Geometry check sheet. Reference: the model listing, model coordinates, mm. Face numbers are marked on the shaded views. A direction names the side the tool comes from. Give positions to 0.01 mm unless a question says otherwise; leave off trailing zeros. Order: outer loops, then holes, each group sorted by start corner. A loop starts at its lowest first (then second) coordinate and runs counter-clockwise, first axis right, second up. Notation, with made-up numbers: M 33,-31 L 78,-31 A21 cw 78,-17 Z; hole C 7.5,89.25 d8. An arc over 180 degrees is marked long. Answer as CSV lines item,"result". Start each with the question number.
Q1. Thickness scan on line 1 (X direction, y = 8, z = 3.75); line 2 (Y direction, x = -21, z = 3.25); line 3 (Y direction, x = -22.25, z = 1.6). Record the ranges inside material, lowest first.
Q2. Set-up check for the marked faces 1, 2, 3, 4 and 5: record each of +Z, -Z, +X, -X, +Y, -Y from which the full face is reachable in a straight line by a thin tool's end or side.
Q3. Section check C-C, the plane y = 9.5. Record the boundary of the cut face in (x, z) (3 decimals), then the cut area to 3 significant figures.
Q4. Section check A-A, the plane z = 2.85. Count the separate pieces of the cut face and the enclosed holes in it, then the cut area to 3 significant figures.
Q5. Section check B-B, the plane x = -19.25. Record the boundary of the cut face in (y, z) (3 decimals).
Q6. Mould release check, pull along X, two halves, no side actions. Record for the marked faces 6, 7 and 8: +X half, -X half, draft (parallel to the pull), parting line (faces both ways), or undercut.
Q7. Go/stop test with flat-tipped pins: pin 1 (0.6 mm diameter, centred on x = -26, z = 3.5, fed in from +Y); pin 2 (1 mm diameter, centred on x = -23.5, z = 3.5, fed in from -Y); pin 3 (1.5 mm diameter, centred on x = -18, y = 14.5, fed in from +Z) (3 decimals). Record where each tip stops, or that it passes through.
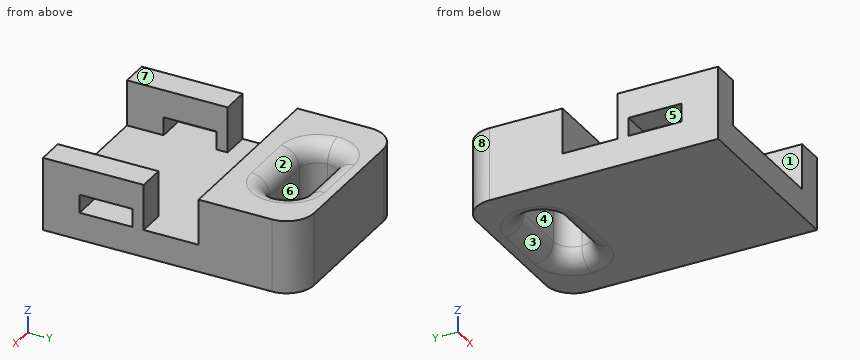
```python
from build123d import *

# Parameters (mm, degrees)
F0_W      = 12.7
F0_H      = 15.24
F1_DEPTH  = 5.08
F2_W      = 6.35
F2_H      = 2.54
F3_DEPTH  = 25.4
F4_R      = 1.26999
F5_R      = 1.905
F6_W      = 5.715
F6_H      = 1.27
F7_DEPTH  = 25.4
F8_W      = 8.89
F8_H      = 8.255
F9_DEPTH  = 3.175
F10_W     = 1.905
F10_H     = 3.81
F11_DEPTH = 1.905
F12_DEPTH = 2.54
F13_W     = 2.5417556653
F13_H     = 1.27
F14_DEPTH = 25.4
F15_W     = 1.905
F15_H     = 0.762
F16_DEPTH = 1.27
F17_W     = 1.905
F17_H     = 0.762
F18_DEPTH = 1.27


# Not quite as in the source:
# - a fillet or chamfer is up to 0.001 mm smaller than in the source, because OpenCascade refuses the exact size


with BuildPart() as f1:
    # F0 (on Top) → F1 (new body)
    with BuildSketch(Plane.XY):
        with Locations((-20.7207803614, 14.9625845535)):
            Rectangle(F0_W, F0_H)
    extrude(amount=F1_DEPTH)

    # F2 (on face) → F3 (cut)
    with BuildSketch(Plane.XY.offset(5.08)):
        with Locations((-20.7207803614, 19.4075845535)):
            Rectangle(F2_W, F2_H)
    extrude(amount=-F3_DEPTH, mode=Mode.SUBTRACT)

    # F4 (radius 1.27 in the source; OpenCascade refuses exactly that, so slightly less here)
    f4_edges = [f1.edges().sort_by_distance(p)[0] for p in [
        (-20.72078, 18.137585, 5.08),
        (-17.54578, 19.407585, 5.08),
        (-23.89578, 19.407585, 5.08),
        (-20.72078, 20.677585, 5.08),
        (-17.54578, 19.407585, 0),
        (-20.72078, 18.137585, 0),
        (-23.89578, 19.407585, 0),
        (-20.72078, 20.677585, 0),
        (-17.54578, 18.137585, 2.54),
        (-23.89578, 18.137585, 2.54),
        (-23.89578, 20.677585, 2.54),
        (-17.54578, 20.677585, 2.54),
    ]]
    fillet(f4_edges, radius=F4_R)

    # F5
    f5_edges = [f1.edges().sort_by_distance(p)[0] for p in [
        (-27.07078, 22.582585, 2.54),
        (-14.37078, 22.582585, 2.54),
    ]]
    fillet(f5_edges, radius=F5_R)

    # F6 (on face) → F7 (cut)
    with BuildSketch(Plane.YZ.offset(-14.3707803614)):
        with Locations((12.7400845535, 2.54)):
            Rectangle(F6_W, F6_H)
    extrude(amount=-F7_DEPTH, mode=Mode.SUBTRACT)

    # F8 (on face) → F9 (cut, through all)
    with BuildSketch(Plane.XY.offset(5.08)):
        with Locations((-20.7207803614, 11.4700845535)):
            Rectangle(F8_W, F8_H)
    extrude(amount=-F9_DEPTH, mode=Mode.SUBTRACT)

    # F10 (on face) → F11 (cut, through all)
    with BuildSketch(Plane.XY.offset(5.08)):
        with Locations((-26.1182803614, 13.6925845535)):
            Rectangle(F10_W, F10_H)
        with Locations((-15.3232803614, 13.6925845535)):
            Rectangle(F10_W, F10_H)
    extrude(amount=-F11_DEPTH, mode=Mode.SUBTRACT)

    # F12 (add): a face of the model
    f12_faces = [f1.faces().sort_by_distance(p)[0] for p in [
        (-20.7207803614, 7.3425845535, 1.7991666667),
    ]]
    extrude(f12_faces, amount=F12_DEPTH)

    # F13 (on face) → F14 (cut)
    with BuildSketch(Plane.YZ.offset(-14.3707803614)):
        with Locations((8.6117067208, 2.54)):
            Rectangle(F13_W, F13_H)
    extrude(amount=-F14_DEPTH, mode=Mode.SUBTRACT)

    # F15 (on face) → F16 (join, through all)
    with BuildSketch(Plane(origin=(0, 0, 3.175), x_dir=(1, 0, 0), z_dir=(0, 0, -1))):
        with Locations((-15.3232803614, -11.4065845535)):
            Rectangle(F15_W, F15_H)
    extrude(amount=F16_DEPTH)

    # F17 (on face) → F18 (join, through all)
    with BuildSketch(Plane(origin=(0, 0, 3.175), x_dir=(1, 0, 0), z_dir=(0, 0, -1))):
        with Locations((-26.1182803614, -11.4065845535)):
            Rectangle(F17_W, F17_H)
    extrude(amount=F18_DEPTH)


solid = f1.part
```
Answer block:
1,line 1,"x = -27.07 to -25.17, -16.28 to -14.37"
1,line 2,"y = 15.6 to 18.14, 20.68 to 22.58"
1,line 3,"y = 4.8 to 18.14, 20.68 to 22.58"
2,face 1,"+Z, -Y"
2,face 2,"+Z"
2,face 3,"-Z"
2,face 4,"+Z, -Z"
2,face 5,"+X, -X"
3,outline,"M -27.071,0 L -14.371,0 L -14.371,1.905 L -27.071,1.905 Z; M -27.071,3.175 L -25.166,3.175 L -25.166,5.08 L -27.071,5.08 Z; M -16.276,3.175 L -14.371,3.175 L -14.371,5.08 L -16.276,5.08 Z"
3,area,"31.5 mm2"
4,separate pieces,"5"
4,enclosed holes,"1"
4,area,"85.0 mm2"
5,outline,"M 4.803,0 L 16.868,0 A1.27 ccw 18.138,1.27 L 18.138,3.81 A1.27 ccw 16.868,5.08 L 15.598,5.08 L 15.598,1.905 L 4.803,1.905 Z; M 20.678,1.27 A1.27 ccw 21.948,0 L 22.583,0 L 22.583,5.08 L 21.948,5.08 A1.27 ccw 20.678,3.81 Z"
6,face 6,"undercut"
6,face 7,"draft"
6,face 8,"-X half"
7,pin 1,"stops at y = 22.51"
7,pin 2,"stops at y = 15.6"
7,pin 3,"stops at z = 1.905"
